For this review, use the dimensioned drawing (mm, ordinates from the lowest corner) and the shaded views. A direction names the side the tool comes from. Give positions to 0.01 mm unless a question says otherwise; leave off trailing zeros.
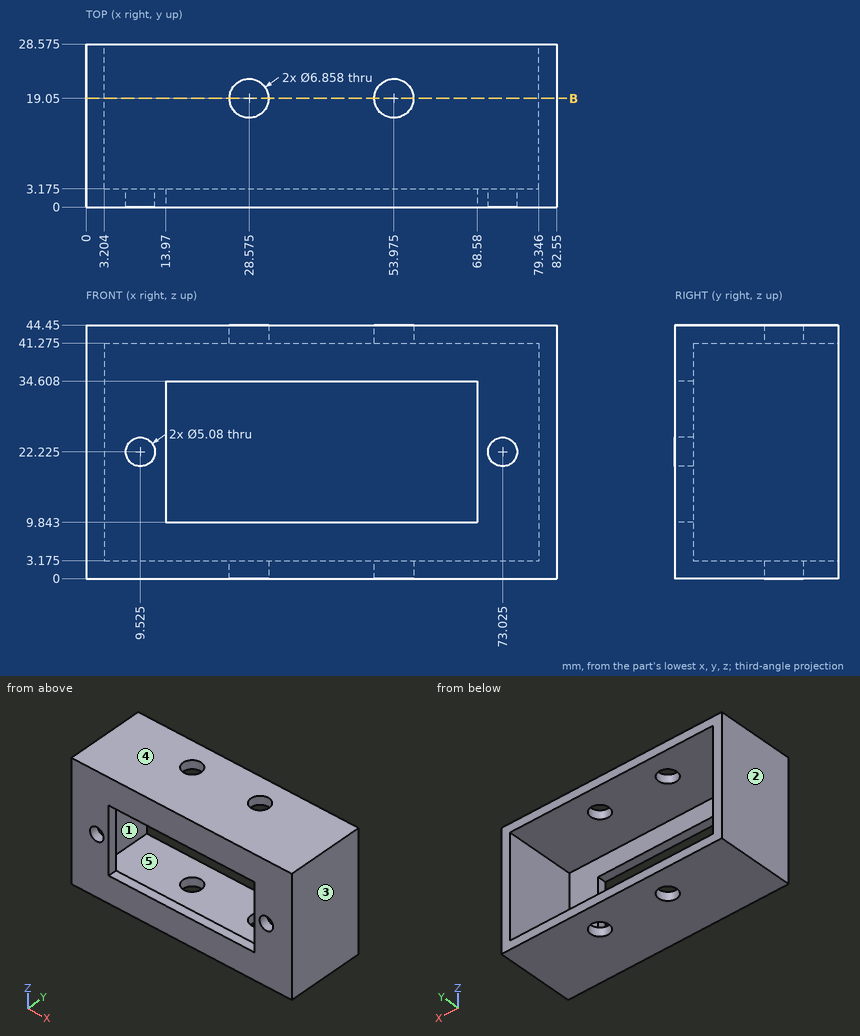
1. Draft analysis for pull direction X (two halves, no side actions). For the marked faces 3, 4 and 5, state which applies: pulls with the +X half, pulls with the -X half, needs draft (parallel to the pull), parting line crosses it, or undercut.
Recorded:
face 3: pulls with the +X half
face 4: needs draft
face 5: undercut
2. Machinability: for the marked faces 1 and 2, which of the approach directions +Z, -Z, +X, -X, +Y, -Y give a long, thin tool a straight path to every point of the face, cutting with its end or side? Answer none if there is none.
Recorded:
face 1: +Y
face 2: +Z, -Z, -X, +Y, -Y
3. For line 1 along Z through (x, y) = (26.5, 2); line 2 along X through (y, z) = (2, 21); line 3 along Y through (x, z) = (77, 4.5) (1 decimal), list the stretches that pass through material, from the lowest coordinate up.
Recorded:
line 1: z = 0 to 9.84, 34.61 to 44.45
line 2: x = 0 to 7.3, 11.75 to 13.97, 68.58 to 70.8, 75.25 to 82.55
line 3: y = 0 to 3.2
4. For pin 1 (4 mm diameter, centred on x = 53.975, y = 19.05, fed in from -Z), flat-tipped, find the tip position at first contact; note if it passes through.
Recorded:
pin 1: passes through
5. Take a section at B-B (y = 19.05). State how many separate pieces and enclosed holes the cut face has.
Recorded:
separate pieces: 4
enclosed holes: 0
